Part print with two shaded views. Sizes in mm from the minimum x, y, z corner. A direction names the side the tool comes from. Give positions to 0.01 mm unless a question says otherwise; leave off trailing zeros. Order: outer loops, then holes, each group sorted by start corner. A loop starts at its lowest first (then second) coordinate and runs counter-clockwise, first axis right, second up. Notation, with made-up numbers: M -18.5,12 L 3.5,12 A23 cw 3.5,20 Z; hole C 70.5,57 d7. An arc over 180 degrees is marked long. Return JSON: item names as keys, results as strings. Group by question number.
1. Pin check, flat tips, straight feed: pin 1 (4 mm diameter, centred on x = 54.5, y = 44.5, fed in from -Z); pin 2 (2 mm diameter, centred on x = 31.5, z = 53, fed in from +Y); pin 3 (2.5 mm diameter, centred on y = 19, z = 55, fed in from +X); pin 4 (8 mm diameter, centred on x = 16.5, y = 107, fed in from +Z). Stop position of each tip, or through.
2. Slice it at B-B on x = 28.5. List the corners of the cut face in (y, z), then the cut area to 3 significant figures.
3. 3-axis set-ups, long thin cutter, end or side, ignore diameter. For the marked faces 1, 2 and 3: which of +Z, -Z, +X, -X, +Y, -Y reach the whole face in a straight line?
4. Slice it at A-A on z = 28.5. List the corners of the cut face in (x, y), then the cut area to 3 significant figures.
5. Slice it at C-C on y = 36.5. List the corners of the cut face in (x, z).
6. Wall check: probe 1 along Z at (x, y) = (28.5, 82.8); probe 2 along Y at (x, z) = (53, 55); probe 3 along Z at (x, y) = (27, 72.5). Give the ranges that are in metal, low to high. Write a range as [from, to].
7. Slice it at D-D on y = 97.5. List the corners of the cut face in (x, z), then the cut area to 3 significant figures.
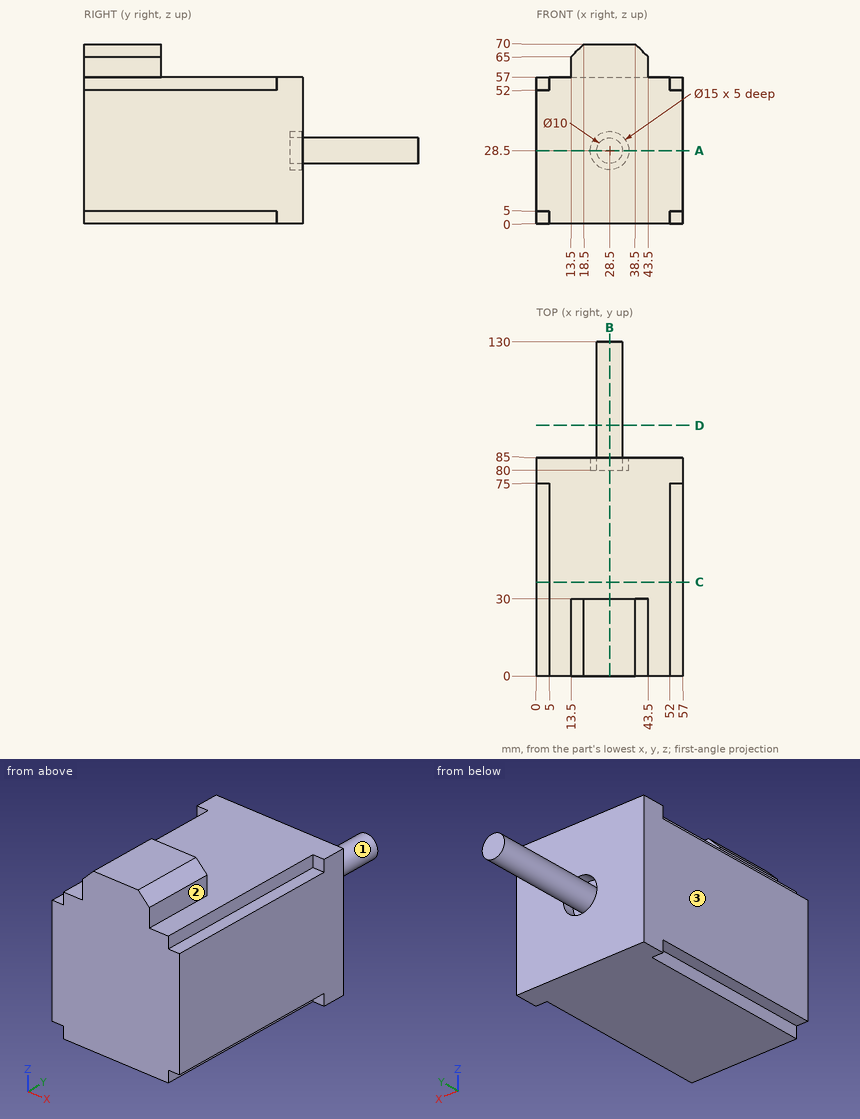
Result:
{
 "1": {"pin 1": "stops at z = 5", "pin 2": "stops at y = 85", "pin 3": "stops at x = 52", "pin 4": "passes through"},
 "2": {"outline": "M 0,0 L 85,0 L 85,21 L 80,21 L 80,23.5 L 130,23.5 L 130,33.5 L 80,33.5 L 80,36 L 85,36 L 85,57 L 30,57 L 30,70 L 0,70 Z", "area": "5,660 mm2"},
 "3": {"face 1": "+Y", "face 2": "+Z, +X, +Y, -Y", "face 3": "+Z, -Z, -X, +Y, -Y"},
 "4": {"outline": "M 0,0 L 57,0 L 57,85 L 36,85 L 36,80 L 33.5,80 L 33.5,130 L 23.5,130 L 23.5,80 L 21,80 L 21,85 L 0,85 Z", "area": "5,270 mm2"},
 "5": {"outline": "M 0,5 L 5,5 L 5,0 L 52,0 L 52,5 L 57,5 L 57,52 L 52,52 L 52,57 L 5,57 L 5,52 L 0,52 Z"},
 "6": {"probe 1": "z = [0, 21], [23.5, 33.5], [36, 57]", "probe 2": "y = [75, 85]", "probe 3": "z = [0, 57]"},
 "7": {"outline": "C 28.5,28.5 d10", "area": "78.5 mm2"}
}
